Check sheet for the modelled part. Datum: model origin and axes. Units: mm. A direction names the side the tool comes from. Coordinates: 2 decimals unless noted, no trailing zeros. Loops run counter-clockwise (first coordinate to the right, second up) from the corner with the lowest first, then second, coordinate; pieces in that order, holes last. Notation, with made-up numbers: M 56,-24 L 88,-24 A34 ccw 88,11 Z; hole C -29,22 d1. An arc over 180 degrees is marked long. Use CSV: the item, a comma, the result in double quotes. Start each with the question number.
(1) Section check B-B on x = -15. Record the cut outline in (y, z).
(2) Go/stop test with flat-tipped pins: pin 1 Ø2 at (x, y) = (-15.5, 1.5) entering from -Z; pin 2 Ø1.4 at (x, y) = (-14.5, 1) entering from -Z; pin 3 Ø2 at (y, z) = (0.5, 50) entering from +X. Record where each tip stops, or that it passes through.
(3) Set-up check for faces 5 (the flat face through (-10.888, -0.03, 38.112)), 6 (the flat face through (-7, -2.15, 26)), 7 (the flat face through (-11.504, 0, 57)), 8 (the flat face through (-7, 2.15, 26)): record each of +Z, -Z, +X, -X, +Y, -Y from which the full face is reachable in a straight line by a thin tool's end or side.
(4) Scan lines: line 1 (Z direction, x = -15.5, y = 1.25); line 2 (Z direction, x = -15, y = -3); line 3 (Y direction, x = -10.25, z = 36). Record each from-to range of solid material in increasing order.
(5) Section check D-D on y = 3. Record the cut outline in (x, z).
(6) Section check A-A on y = 0.5. Record the cut outline in (x, z), and give its area (3 significant figures).
(7) Draft check along Z on faces 1 (the flat face through (-7.704, 0, 15)), 2 (the flat face through (-12.01, 0.03, 52.95)), 3 (the flat face through (-15.704, 0, 49)), 4 (the flat face through (-12.52, -0.03, 37.94)). Enter one of: pulls with the +Z half, pulls with the -Z half, needs draft (parallel to the pull), parting line crosses it, or undercut.
(8) Section check C-C on z = 7. Record the cut outline in (x, y), and give its area (3 significant figures).
from build123d import *

# Parameters (mm, degrees)
F1_DEPTH = 2.15
F2_W     = 5.7
F2_H     = 7.6
F3_DEPTH = 1.65
F5_DEPTH = 1.6
F6_SIZE  = 1


with BuildPart() as f1:
    # F0 (on Front) → F1 (new body, symmetric)
    with BuildSketch(Plane.XZ):
        Polygon((-7.7040915435, 0), (-6.2040915435, 0), (-6.2040915435, 30), (-15.7040915435, 46.4544826719), (-15.7040915435, 52.4544826719), (-11.5040915435, 52.4544826719), (-11.5040915435, 60.0544826719), (-17.2040915435, 60.0544826719), (-17.2040915435, 46.0525588833), (-7.7040915435, 29.5980762114), align=None)
    extrude(amount=F1_DEPTH, both=True)

    # F2 (on face) + F1_face1 (on face) → F3 (join)
    with BuildSketch(Plane.XZ.offset(2.15)):
        with Locations((-14.3540915435, 56.2544826719)):
            Rectangle(F2_W, F2_H)
    with BuildSketch(Plane(origin=(-11.28016615, 2.15, 36.9237290057), x_dir=(1, 0, 0), z_dir=(0, 1, 0))):
        Polygon((5.0760746065, 36.9237290057), (3.5760746065, 36.9237290057), (3.5760746065, 7.3256527943), (-5.9239253935, -9.1288298776), (-5.9239253935, -23.1307536662), (-0.2239253935, -23.1307536662), (-0.2239253935, -15.5307536662), (-4.4239253935, -15.5307536662), (-4.4239253935, -9.5307536662), (5.0760746065, 6.9237290057), align=None)
    extrude(amount=F3_DEPTH, dir=(0, -1, 0))

    # F4 (on face) → F5 (join)
    with BuildSketch(Plane(origin=(0, 2.15, 0), x_dir=(-1, 0, 0), z_dir=(0, 1, 0))):
        Polygon((17.2040915435, 52.4544826719), (17.2040915435, 60.0544826719), (11.5040915435, 60.0544826719), (11.5040915435, 52.4544826719), (15.7040915435, 52.4544826719), align=None)
    extrude(amount=F5_DEPTH)

    # F6
    f6_edges = [f1.edges().sort_by_distance(p)[0] for p in [
        (-11.504092, -0.025, 52.454483),
    ]]
    chamfer(f6_edges, length=F6_SIZE)


solid = f1.part
Outcome:
1,outline,"M -3.8,52.45 L 3.75,52.45 L 3.75,60.05 L -3.8,60.05 Z; M -2.15,42.23 L 2.15,42.23 L 2.15,45.23 L -2.15,45.23 Z"
2,pin 1,"stops at z = 41.37"
2,pin 2,"stops at z = 40.16"
2,pin 3,"stops at x = -15.7"
3,face 5,"+X, +Y, -Y"
3,face 6,"-Z, +X, -X, -Y"
3,face 7,"+Z, +X, +Y, -Y"
3,face 8,"-Z, +X, -X, +Y"
4,line 1,"z = 43.1 to 46.1, 52.45 to 60.05"
4,line 2,"z = 52.45 to 60.05"
4,line 3,"y = -2.15 to 2.15"
5,outline,"M -17.2,52.45 L -12.5,52.45 L -11.5,53.45 L -11.5,60.05 L -17.2,60.05 Z"
6,outline,"M -17.2,46.05 L -7.7,29.6 L -7.7,0 L -6.2,0 L -6.2,30 L -15.7,46.45 L -15.7,52.45 L -12.5,52.45 L -11.5,53.45 L -11.5,60.05 L -17.2,60.05 Z"
6,area,"125 mm²"
7,face 1,"needs draft"
7,face 2,"undercut"
7,face 3,"undercut"
7,face 4,"pulls with the -Z half"
8,outline,"M -7.7,-2.15 L -6.2,-2.15 L -6.2,2.15 L -7.7,2.15 Z"
8,area,"6.45 mm²"
